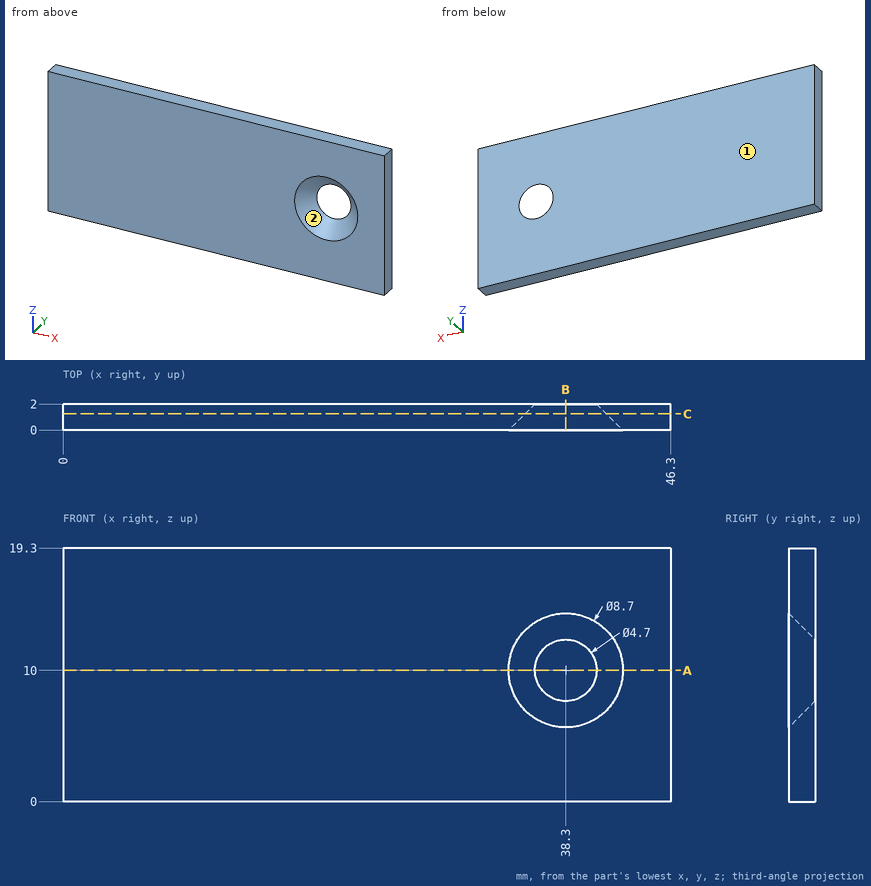
Part print with two shaded views. Sizes in mm from the minimum x, y, z corner. Give positions to 0.01 mm unless a question says otherwise; leave off trailing zeros. Loops run counter-clockwise (first coordinate to the right, second up) from the corner with the lowest first, then second, coordinate; pieces in that order, holes last. Notation, with made-up numbers: (10, 73) -> (28, 73) arc R28 cw to (28, 95) -> close; hole circle Ø7 at (-10.5, -14.75). An arc over 180 degrees is marked (long way). One line per question, with ' | ' between items.
Q1. Drill centre lines: line 1 along Z through (x, y) = (36, 0.5); line 2 along X through (y, z) = (0.5, 8.25); line 3 along Y through (x, z) = (39, 13). Where is each one in solid material? Low to high. Write a range as [from, to].
Filled sheet:
line 1: z = [0, 6.91], [13.09, 19.3] | line 2: x = [0, 34.87], [41.73, 46.3] | line 3: y = [1.27, 2]
Q2. Cut at A-A, the plane z = 10. Write the cut outline in (x, y).
Filled sheet:
outline: (0, 0) -> (33.95, 0) -> (35.95, 2) -> (0, 2) -> close; (40.65, 2) -> (42.65, 0) -> (46.3, 0) -> (46.3, 2) -> close
Q3. Cut at B-B, the plane x = 38.3. Write the cut outline in (y, z).
Filled sheet:
outline: (0, 0) -> (2, 0) -> (2, 7.65) -> (0, 5.65) -> close; (0, 14.35) -> (2, 12.35) -> (2, 19.3) -> (0, 19.3) -> close
Q4. Cut at C-C, the plane y = 1.25. Write the cut outline in (x, z).
Filled sheet:
outline: (0, 0) -> (46.3, 0) -> (46.3, 19.3) -> (0, 19.3) -> close; hole circle Ø6.2 at (38.3, 10)
Q5. Pull direction Z, two halves, no side cores. Call the marked faces 1 and 2: pulls with the +Z half, pulls with the -Z half, needs draft (parallel to the pull), parting line crosses it, or undercut.
Filled sheet:
face 1: needs draft | face 2: undercut
